Autodesk Inventor part; units mm, degrees
ref_plane "YZ Plane" through (0, 0, 0) normal (1, 0, 0) x (0, 1, 0)
ref_plane "XZ Plane" through (0, 0, 0) normal (0, 1, 0) x (-1, 0, 0)
ref_plane "XY Plane" through (0, 0, 0) normal (0, 0, 1) x (1, 0, 0)
sketch "Sketch1" plane through (0, 0, 0) normal (0, 0, 1) x (1, 0, 0)
  circle A0 centre (0, 0) radius 12.7
  dimension "d0" = 25.4
extrude "Extrusion1" add sketch "Sketch1" along normal blind 69.85
sketch "Sketch2" plane through (0, 0, 69.85) normal (0, 0, 1) x (1, 0, 0)
  circle A0 centre (0, 0) radius 7.9375
  dimension "d3" = 15.875
extrude "Extrusion2" cut sketch "Sketch2" against normal blind 45.72
sketch "Sketch3" plane through (0, 0, 24.13) normal (0, 0, 1) x (1, 0, 0)
  point P0 (0, 0)
  point P1 (0, 0)
hole "Hole1" at (0, 0, 24.13) direction (0, 0, -1) diameter 10.5918 end through all
chamfer "Chamfer1" distance 2.54 angle 45 1 edges at (-12.7, 0, 69.85)
properties part number "Top_attachment"
Check sheet for the modelled part. Datum: model origin and axes. Units: mm. A direction names the side the tool comes from. Give positions to 0.01 mm unless a question says otherwise; leave off trailing zeros. Write each loop counter-clockwise with the first axis right and the second up, starting at its lowest first coordinate (ties: lowest second). Pieces come first, ordered by that corner, then holes.
Item 1: Gauge pin test, flat ends, axial feed: pin 1 (4 mm diameter, centred on x = -9.5, y = -9.5, fed in from +Z) (3 decimals); pin 2 (2 mm diameter, centred on x = -9.5, z = 36.5, fed in from -Y); pin 3 (12 mm diameter, centred on x = 10, z = 22, fed in from +Y). Record the tip position at first contact, or that the pin passes through.
Item 2: Cross-section at A-A (y = 0). Enter the section's corners in (x, z).
Item 3: Draft check along Y on faces 1 (the face through (-2.237, 10.074, 69.691)), 2 (the face through (5.17, 1.15, 11.9)), 3 (the face through (-6.8, -4.5, 69.85)), 4 (the face through (-1.72, -7.75, 47.31)). Enter one of: released by +Y, released by -Y, zero draft, split by the parting line, or undercut.
Item 4: Cross-section at C-C (z = 34.5). Enter the section's corners in (x, y) (1 decimal).
Item 5: Access from +Z, -Z, +X, -X, +Y, -Y to the whole of each face (thin tool, end or side, straight path). Record for faces 5 (the face through (5.2, -1.7, 24.13)), 6 (the face through (-2.75, 12.4, 33.18)).
Item 6: Scan lines: L1, parallel to Y at x = 0, z = 38; L2, parallel to Y at x = 0, z = 19; L3, parallel to X at y = -0.5, z = 45.5. Record each from-to range of solid material in increasing order.
Report:
1. pin 1: stops at z = 68.575
1. pin 2: stops at y = -9.44
1. pin 3: stops at y = 12.05
2. outline: (-12.7, 0) - (-5.3, 0) - (-5.3, 24.13) - (-7.94, 24.13) - (-7.94, 69.85) - (-10.16, 69.85) - (-12.7, 67.31) - close; (5.3, 0) - (12.7, 0) - (12.7, 67.31) - (10.16, 69.85) - (7.94, 69.85) - (7.94, 24.13) - (5.3, 24.13) - close
3. face 1: split by the parting line
3. face 2: undercut
3. face 3: zero draft
3. face 4: undercut
4. outline: circle Ø25.4 at (0, 0); hole circle Ø15.9 at (0, 0)
5. face 5: +Z
5. face 6: +Z, -Z
6. L1: y = -12.7 to -7.94, 7.94 to 12.7
6. L2: y = -12.7 to -5.3, 5.3 to 12.7
6. L3: x = -12.69 to -7.92, 7.92 to 12.69
